from build123d import *

# Parameters (mm, degrees)
F0_W           = 406
F0_H           = 12.7
F1_DEPTH       = 9.55
F3_D           = 4.4
F3_DEPTH       = 20
F3_CBORE_D     = 8.25
F3_CBORE_DEPTH = 4
F3_TIP         = 1.3218933619
F5_D           = 4.4


with BuildPart() as f1:
    # F0 (on Top) → F1 (new body, symmetric)
    with BuildSketch(Plane.XY):
        Rectangle(F0_W, F0_H)
    extrude(amount=F1_DEPTH, both=True)

    # F3
    with Locations(Plane.XY.offset(9.55)):
        with Locations((-198.2, 0), (-188.7, 0), (188.7, 0), (198.2, 0)):
            CounterBoreHole(F3_D / 2, F3_CBORE_D / 2, F3_CBORE_DEPTH, depth=F3_DEPTH)
            with Locations((0, 0, -(F3_DEPTH + F3_TIP / 2))):  # 118° drill point
                Cone(0, F3_D / 2, F3_TIP, mode=Mode.SUBTRACT)

    # F5 (through all)
    with Locations(Plane.XY.offset(9.55)):
        with Locations((-171, 0), (-152, 0), (-133, 0), (-114, 0), (-95, 0), (-57, 0), (-38, 0), (-76, 0), (-19, 0), (0, 0), (19, 0), (38, 0), (57, 0), (76, 0), (95, 0), (114, 0), (133, 0), (152, 0), (171, 0), (133, 0)):
            Hole(F5_D / 2)


solid = f1.part
Geometry check sheet. Reference: the model listing, model coordinates, mm. A direction names the side the tool comes from. Give positions to 0.01 mm unless a question says otherwise; leave off trailing zeros. Answer as a JSON object with one key per item and string values.
(1) Draft check along Y on faces 1 (the flat face through (-3, -6.35, 0)), 2 (the flat face through (-203, 0, 0)), 3 (the flat face through (-196, -2, 5.55)). Enter one of: released by +Y, released by -Y, zero draft, split by the parting line, or undercut.
Report:
{"face 1": "released by -Y", "face 2": "zero draft", "face 3": "undercut"}
(2) Tool access check on faces 4 (the flat face through (190, -2, 5.55)), 5 (the flat face through (-3, 0, -9.55)). Record the directions out of +Z, -Z, +X, -X, +Y, -Y that give a thin tool (end or side, any length) a straight path to the whole face; none if there is none.
Report:
{"face 4": "+Z", "face 5": "-Z, +X, -X, +Y, -Y"}
(3) Material ranges on line 1 (Y direction, x = 38, z = -3.75); line 2 (Y direction, x = 40, z = -7.5), recorded low to high.
Report:
{"line 1": "-6.35 to -2.2, 2.2 to 6.35", "line 2": "-6.35 to -0.92, 0.92 to 6.35"}
(4) Cross-section at A-A (z = 0). State how many separate pieces and enclosed holes the cut face has, then the cut area to 3 significant figures.
Report:
{"separate pieces": "1", "enclosed holes": "23", "area": "4,810 mm^2"}
